from build123d import *

# Parameters (mm, degrees)
SKETCH1_W               = 3.5
SKETCH1_H               = 15.967998052
BOSS_EXTRUDE1_DEPTH     = 19
BOSS_EXTRUDE2_START     = 27
SKETCH2_R               = 6.5
SKETCH2_R_2             = 2
BOSS_EXTRUDE2_DEPTH     = 5
BOSS_EXTRUDE3_DEPTH     = 97.75
FILLET1_START           = -72
FILLET1_DEPTH           = 99
CUT_EXTRUDE1_DEPTH      = 85.442658059
CUT_EXTRUDE1_DEPTH_BACK = 85.442658059
SKETCH4_R               = 3
CHAMFER1_SIZE           = 4
FILLET3_R               = 4


with BuildPart() as part:
    # Sketch1 → Boss-Extrude1 (new body)
    with BuildSketch(Plane.XY):
        Polygon((-59.25, 0), (59.25, 0), (59.25, -20), (70.75, -20), (70.75, 4), (-70.75, 4), (-70.75, -20), (-59.25, -20), align=None)
        with Locations((65, -8.016000974)):
            Rectangle(SKETCH1_W, SKETCH1_H, mode=Mode.SUBTRACT)
        with Locations((-65, -8.016000974)):
            Rectangle(SKETCH1_W, SKETCH1_H, mode=Mode.SUBTRACT)
    extrude(amount=-BOSS_EXTRUDE1_DEPTH)

    # Sketch2 → Boss-Extrude2 (add)
    with BuildSketch(Plane(origin=(0, 0, 0), x_dir=(0, 0, -1), z_dir=(1, 0, 0)).offset(BOSS_EXTRUDE2_START)):
        with BuildLine():
            Line((19, 4), (19, 23))
            ThreePointArc((19, 23), (-13.435028843, 36.435028843), (0, 4))
            Line((0, 4), (19, 4))
        make_face()
        with Locations((0, 30)):
            Circle(SKETCH2_R, mode=Mode.SUBTRACT)
        with Locations((15.5, 23)):
            Circle(SKETCH2_R_2, mode=Mode.SUBTRACT)
        with Locations((7.75, 9.576606241)):
            Circle(SKETCH2_R_2, mode=Mode.SUBTRACT)
        with Locations((-7.75, 9.576606241)):
            Circle(SKETCH2_R_2, mode=Mode.SUBTRACT)
        with Locations((-15.5, 23)):
            Circle(SKETCH2_R_2, mode=Mode.SUBTRACT)
        with Locations((-7.75, 36.423393759)):
            Circle(SKETCH2_R_2, mode=Mode.SUBTRACT)
        with Locations((7.75, 36.423393759)):
            Circle(SKETCH2_R_2, mode=Mode.SUBTRACT)
    extrude(amount=BOSS_EXTRUDE2_DEPTH)

    # Sketch3 → Boss-Extrude3 (add)
    with BuildSketch(Plane.ZY.offset(70.75)):
        with BuildLine():
            Line((0, 4), (-19, 4))
            Line((-19, 4), (-19, 23))
            ThreePointArc((-19, 23), (-13.435028843, 9.564971157), (0, 4))
        make_face()
    extrude(amount=-BOSS_EXTRUDE3_DEPTH)

    # Fillet1: read off the stored shape, not the designer's step
    # Fillet1 outline → Fillet1 (cut)
    with BuildSketch(Plane.YZ.offset(FILLET1_START)):
        with BuildLine():
            ThreePointArc((23, -19), (19.957565078, -18.754828438), (16.993647895, -18.025641026))
            ThreePointArc((16.993647895, -18.025641026), (17.329134114, -18.580064077), (16.835585997, -19))
            Line((16.835585997, -19), (23, -19))
        make_face()
    extrude(amount=FILLET1_DEPTH, mode=Mode.SUBTRACT)

    # Sketch4 → Cut-Extrude1 (cut, two sides: drawn at the far end of the back side and taken through both)
    with BuildSketch(Plane(origin=(0, 0, 0), x_dir=(0, 0, -1), z_dir=(1, 0, 0)).offset(-CUT_EXTRUDE1_DEPTH_BACK)):
        with Locations((9.246961263, -10.5)):
            Circle(SKETCH4_R)
    extrude(amount=CUT_EXTRUDE1_DEPTH + CUT_EXTRUDE1_DEPTH_BACK, mode=Mode.SUBTRACT)

    # Chamfer1
    # the kernel refuses this chamfer: 4 mm, written as the material it adds along each edge
    with BuildSketch(Plane(origin=(27, 4, 0), x_dir=(0, -1, 0), z_dir=(1, 0, 0))) as chamfer1_piece_1:
        with BuildLine():
            Line((CHAMFER1_SIZE, 0), (-0.553778005, -4.553778005))
            ThreePointArc((-0.553778005, -4.553778005), (-0.146737714, -2.356798922), (0, 0))
            Line((0, 0), (CHAMFER1_SIZE, 0))
        make_face()
    extrude(amount=5)

    # Fillet3
    fillet3_edges = [part.edges().sort_by_distance(p)[0] for p in [
        (59.25, -20, -9.5),
        (-59.25, -20, -9.5),
        (-70.75, -20, -9.5),
        (70.75, -20, -9.5),
    ]]
    fillet(fillet3_edges, radius=FILLET3_R)


solid = part.part
Can you work these out from the model? Positions are in its coordinate system, mm. A direction names the side the tool comes from. Coordinates: 2 decimals unless noted, no trailing zeros. Order: outer loops, then holes, each group sorted by start corner. A loop starts at its lowest first (then second) coordinate and runs counter-clockwise, first axis right, second up. Notation, with made-up numbers: M 56.25,84 L 80.25,84 A26 ccw 80.25,106 Z; hole C 77,-26 d8. An arc over 180 degrees is marked long. Answer as CSV lines item,"result".
(1) Suppose I cut it at A-A on y = -5.5. Please give me the cut outline in (x, z).
Geometry check:
outline,"M -70.75,-19 L -66.75,-19 L -66.75,0 L -70.75,0 Z; M -63.25,-19 L -59.25,-19 L -59.25,0 L -63.25,0 Z; M 59.25,-19 L 63.25,-19 L 63.25,0 L 59.25,0 Z; M 66.75,-19 L 70.75,-19 L 70.75,0 L 66.75,0 Z"
(2) If we mould it in two halves opening along Z, with no side actions, what happens to faces 6 (the cylindrical face through (29.465, 38.406, 8.01)), 7 (the flat face through (-59.25, -6, -9)), 8 (the flat face through (29, 2, 2))? For each: released by +Z, released by -Z, zero draft, split by the parting line, or undercut.
Geometry check:
face 6,"undercut"
face 7,"zero draft"
face 8,"released by +Z"
(3) Suppose I cut it at D-D on y = 26.5. Please give me the cut outline in (x, z), plus the area to 3 significant figures.
Geometry check:
outline,"M 27,-18.67 L 32,-18.67 L 32,-5.48 L 27,-5.48 Z; M 27,5.48 L 32,5.48 L 32,18.67 L 27,18.67 Z"
area,"132 mm^2"
(4) I'm going to push flat-ended pins straight in: pin 1 (15 mm diameter, centred on x = 49, z = -11, fed in from +Y); pin 2 (2.5 mm diameter, centred on y = 23, z = 15.5, fed in from +X); pin 3 (12 mm diameter, centred on x = -16, y = -2, fed in from +Z); pin 4 (3 mm diameter, centred on x = -27.5, z = -4.5, fed in from -Y). Where does each tip first touch, or does it pass through?
Geometry check:
pin 1,"y = 4"
pin 2,"through"
pin 3,"z = 0"
pin 4,"y = 0"
(5) Suppose I cut it at B-B on z = -15. Please give me the cut outline in (x, y), plus the area to 3 significant figures.
Geometry check:
outline,"M -70.75,-16 A4 ccw -66.75,-20 L -63.25,-20 A4 ccw -59.25,-16 L -59.25,0 L 59.25,0 L 59.25,-16 A4 ccw 63.25,-20 L 66.75,-20 A4 ccw 70.75,-16 L 70.75,4 L 32,4 L 32,21.06 L 27,21.06 L 27,11.34 L -70.75,11.34 Z; M 27,24.94 L 32,24.94 L 32,34.66 L 27,34.66 Z; hole M -66.75,-16 L -63.25,-16 L -63.25,-0.03 L -66.75,-0.03 Z; hole M 63.25,-16 L 66.75,-16 L 66.75,-0.03 L 63.25,-0.03 Z"
area,"1,750 mm^2"
(6) Suppose I cut it at C-C on x = -28. Please give me the cut outline in (y, z), plus the area to 3 significant figures.
Geometry check:
outline,"M 0,-19 L 16.84,-19 A0.5 ccw 16.99,-18.03 A19 cw 4,0 L 0,0 Z"
area,"152 mm^2"
(7) On a 3-axis mill with a long thin cutter (end or side, diameter ignored), from which of +Z, -Z, +X, -X, +Y, -Y can I reach the whole of each face in a straight line? I mean faces 1 (the flat face through (66.75, -6, -9)), 2 (the flat face through (65, -20, -9)), 3 (the cylindrical face through (-22.56, 7.68, -11.24)), 4 (the flat face through (60, -2, 0)), 5 (the cylindrical face through (29.465, 38.406, -7.49)). Say none if no direction works.
Geometry check:
face 1,"+Z, -Z"
face 2,"+Z, -Z, +X, -X, -Y"
face 3,"+Z, -X, +Y"
face 4,"+Z, +X, +Y, -Y"
face 5,"+X, -X"
(8) Please list where these lines run through material, in increasing order: L1, parallel to X at y = -6.5, z = -8.5; L2, parallel to Z at x = -62.1, y = -10.5; L3, parallel to Y at x = 28.4, z = -7.75.
Geometry check:
L1,"-70.75 to -66.75, -63.25 to -59.25, 59.25 to 63.25, 66.75 to 70.75"
L2,"-19 to -12.25, -6.25 to 0"
L3,"0 to 7.58, 11.58 to 34.42, 38.42 to 40.35"
